from build123d import *

# Parameters (mm, degrees)
SKETCH1_W           = 29
SKETCH1_H           = 24
BOSS_EXTRUDE1_DEPTH = 2
SKETCH2_W           = 29
SKETCH2_H           = 24
SKETCH2_W_2         = 25
SKETCH2_H_2         = 20
BOSS_EXTRUDE2_DEPTH = 5
SKETCH3_W           = 10
SKETCH3_H           = 2.5
CUT_EXTRUDE1_DEPTH  = 2
SKETCH7_R           = 1
CUT_EXTRUDE2_DEPTH  = 0.5
CUT_EXTRUDE4_DEPTH  = 0.5
FILLET3_R           = 2
FILLET4_R           = 0.5


with BuildPart() as part:
    # Sketch1 → Boss-Extrude1 (new body)
    with BuildSketch(Plane(origin=(0, 0, 0), x_dir=(1, 0, 0), z_dir=(0, 1, 0))):
        Rectangle(SKETCH1_W, SKETCH1_H)
    extrude(amount=BOSS_EXTRUDE1_DEPTH)

    # Sketch2 → Boss-Extrude2 (add)
    with BuildSketch(Plane.XZ):
        Rectangle(SKETCH2_W, SKETCH2_H)
        Rectangle(SKETCH2_W_2, SKETCH2_H_2, mode=Mode.SUBTRACT)
    extrude(amount=BOSS_EXTRUDE2_DEPTH)

    # Sketch3 → Cut-Extrude1 (cut)
    with BuildSketch(Plane(origin=(0, 2, 0), x_dir=(1, 0, 0), z_dir=(0, 1, 0))):
        with Locations((0, 5.75)):
            Rectangle(SKETCH3_W, SKETCH3_H)
    extrude(amount=-CUT_EXTRUDE1_DEPTH, mode=Mode.SUBTRACT)

    # Sketch7 → Cut-Extrude2 (cut)
    with BuildSketch(Plane(origin=(0, 2, 0), x_dir=(1, 0, 0), z_dir=(0, 1, 0))):
        with BuildLine():
            Line((5, -2), (8.464101615, 0))
            Line((8.464101615, 0), (5, 2))
            Line((5, 2), (5, 1))
            Line((5, 1), (1.732050808, 1))
            ThreePointArc((1.732050808, 1), (-1.414213562, 1.414213562), (-1, -1.732050808))
            Line((-1, -1.732050808), (-1, -5))
            Line((-1, -5), (-2, -5))
            Line((-2, -5), (0, -8.464101615))
            Line((0, -8.464101615), (2, -5))
            Line((2, -5), (1, -5))
            Line((1, -5), (1, -1.732050808))
            ThreePointArc((1, -1.732050808), (1.414213562, -1.414213562), (1.732050808, -1))
            Line((1.732050808, -1), (5, -1))
            Line((5, -1), (5, -2))
        make_face()
        with Locations(Location((0, 0, 0), (0, 0, 270))):
            Circle(SKETCH7_R, mode=Mode.SUBTRACT)
    extrude(amount=-CUT_EXTRUDE2_DEPTH, mode=Mode.SUBTRACT)

    # Sketch10 → Cut-Extrude4 (cut)
    with BuildSketch(Plane(origin=(0, 2, 0), x_dir=(1, 0, 0), z_dir=(0, 1, 0))):
        Polygon((9.565905449, 1.057692308), (10.194811699, 1.057692308), (10.893129006, -0.587840545), (11.665765224, 1.057692308), (12.304487179, 1.057692308), (10.660356571, -2.442307692), (10.021634615, -2.442307692), (10.562199519, -1.291766827), align=None)
        Polygon((3.628305288, -6.442307692), (4.337139423, -6.442307692), (4.842648237, -7.139222756), (5.346053686, -6.442307692), (6.056290064, -6.442307692), (5.198818109, -7.630008013), (6.192307692, -9), (5.483473558, -9), (4.844751603, -8.120092147), (4.209535256, -9), (3.5, -9), (4.489282853, -7.629306891), align=None)
        Polygon((-4.775641026, 1.057692308), (-2.801282051, 1.057692308), (-3.977063301, -0.961538462), (-2.891025641, -0.961538462), (-2.891025641, -1.5), (-4.955128205, -1.5), (-3.780048077, 0.519230769), (-4.775641026, 0.519230769), align=None)
    extrude(amount=-CUT_EXTRUDE4_DEPTH, mode=Mode.SUBTRACT)

    # Fillet3
    fillet3_edges = [part.edges().sort_by_distance(p)[0] for p in [
        (12.5, -2.5, 10),
        (-12.5, -2.5, 10),
        (-12.5, -2.5, -10),
        (12.5, -2.5, -10),
        (14.5, -1.5, 12),
        (-14.5, -1.5, 12),
        (-14.5, -1.5, -12),
        (14.5, -1.5, -12),
    ]]
    fillet(fillet3_edges, radius=FILLET3_R)

    # Fillet4
    fillet4_edges = [part.edges().sort_by_distance(p)[0] for p in [
        (5, 1, -4.5),
        (5, 1, -7),
        (-5, 1, -7),
        (-5, 1, -4.5),
    ]]
    fillet(fillet4_edges, radius=FILLET4_R)


solid = part.part
Input: part model. Units: mm. Frame: model coordinates. A direction names the side the tool comes from. Give positions to 0.01 mm unless a question says otherwise; leave off trailing zeros. Loops run counter-clockwise (first coordinate to the right, second up) from the corner with the lowest first, then second, coordinate; pieces in that order, holes last. Notation, with made-up numbers: (-36, 57) - (-6, 57) arc R26 ccw to (-6, 73) - close; hole circle Ø3 at (-11, 63). An arc over 180 degrees is marked (long way). Use CSV: the item, a comma, the result in double quotes. Start each with the question number.
Item 1: Contact query for a flat-ended pin moving along its axis: P1, Ø1.5, axis at x = -11.5, z = -1, coming from the -Y side. Output: stop coordinate, or through.
Item 2: Reachability of faces 1 (the cylindrical face through (-11.9, -2.54, 9.43)), 2 (the flat face through (6.756, 1.754, -0.986)), 3 (the cylindrical face through (-13.93, -1.55, -11.4)) from +Z, -Z, +X, -X, +Y, -Y: full face, straight path, thin tool, end or side. Return the list, or none.
Item 3: Mould query, pull axis Z, two halves, no side actions, for faces 4 (the flat face through (0, -1, -12)), 5 (the flat face through (0, 0, 0)), 6 (the flat face through (-14.5, -1, 0)), 7 (the flat face through (6.708, 1.754, 1.014)). Classes: pulls with the +Z half, pulls with the -Z half, needs draft (parallel to the pull), parting line crosses it, or undercut.
Item 4: Section C-C on y = -4. Return loops of the section in (x, z), then the cut area to 3 significant figures.
Item 5: Section D-D on z = -8.5. Return loops of the section in (x, y).
Item 6: Section A-A on x = -9.75. Return loops of the section in (y, z), then the cut area to 3 significant figures.
Item 7: Line query: line 1 (Z direction, x = 2.5, y = -2.5); line 2 (X direction, y = -3.25, z = -2.25); line 3 (Y direction, x = -1.25, z = 5.5). Output: solid intervals per line, ascending.
Item 8: Section B-B on y = 0.75. Return loops of the section in (x, z).
Ans:
1,P1,"stops at y = 0"
2,face 1,"-Y"
2,face 2,"+Y"
2,face 3,"-Z, -X, +Y, -Y"
3,face 4,"pulls with the -Z half"
3,face 5,"undercut"
3,face 6,"needs draft"
3,face 7,"undercut"
4,outline,"(-14.5, -10) arc R2 ccw to (-12.5, -12) - (12.5, -12) arc R2 ccw to (14.5, -10) - (14.5, 10) arc R2 ccw to (12.5, 12) - (-12.5, 12) arc R2 ccw to (-14.5, 10) - close; hole (-12.5, -8) arc R2 ccw to (-10.5, -10) - (10.5, -10) arc R2 ccw to (12.5, -8) - (12.5, 8) arc R2 ccw to (10.5, 10) - (-10.5, 10) arc R2 ccw to (-12.5, 8) - close"
4,area,"196 mm2"
5,outline,"(-14.5, -5) - (-12.44, -5) - (-12.44, 0) - (12.44, 0) - (12.44, -5) - (14.5, -5) - (14.5, 2) - (-14.5, 2) - close"
6,outline,"(-5, -12) - (2, -12) - (2, 12) - (-5, 12) - (-5, 10) - (0, 10) - (0, -10) - (-5, -10) - close"
6,area,"68.0 mm2"
7,line 1,"z = -12 to -10, 10 to 12"
7,line 2,"x = -14.5 to -12.5, 12.5 to 14.5"
7,line 3,"y = 0 to 1.5"
8,outline,"(-14.5, -10) arc R2 ccw to (-12.5, -12) - (12.5, -12) arc R2 ccw to (14.5, -10) - (14.5, 10) arc R2 ccw to (12.5, 12) - (-12.5, 12) arc R2 ccw to (-14.5, 10) - close; hole (-5, -6.5) arc R0.5 ccw to (-4.5, -7) - (4.5, -7) arc R0.5 ccw to (5, -6.5) - (5, -5) arc R0.5 ccw to (4.5, -4.5) - (-4.5, -4.5) arc R0.5 ccw to (-5, -5) - close"
